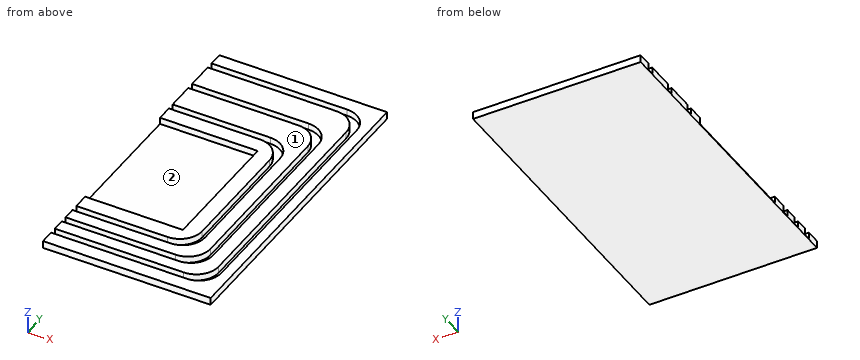
Autodesk Inventor part; units mm, degrees
ref_plane "YZ Plane" through (0, 0, 0) normal (1, 0, 0) x (0, 1, 0)
sketch "Sketch1" plane through (0, 0, 0) normal (0, 0, 1) x (1, 0, 0)
  line L0 (0, -9.3) -> (385, -9.3)
  line L1 (400, -24.3) -> (400, -185)
  line L2 (385, -200) -> (-400, -200)
  line L3 (-400, -200) -> (-400, -32.4)
  line L4 (0, -9.3) -> (0, -13.8)
  line L5 (0, -13.8) -> (380.5, -13.8)
  line L6 (395.5, -28.8) -> (395.5, -180.5)
  line L7 (380.5, -195.5) -> (-395.5, -195.5)
  line L8 (-400, -32.4) -> (372.25, -32.4)
  line L9 (387.25, -47.4) -> (387.25, -172.25)
  line L10 (372.25, -187.25) -> (-387.25, -187.25)
  line L11 (-395.5, -195.5) -> (-395.5, -36.9)
  line L12 (-395.5, -36.9) -> (367.75, -36.9)
  line L13 (382.75, -51.9) -> (382.75, -167.75)
  line L14 (367.75, -182.75) -> (-382.75, -182.75)
  line L15 (-382.75, -182.75) -> (-382.75, -60)
  line L16 (-387.25, -187.25) -> (-387.25, -55.5)
  line L17 (-387.25, -55.5) -> (359.5, -55.5)
  line L18 (374.5, -70.5) -> (374.5, -159.5)
  line L19 (-382.75, -60) -> (355, -60)
  line L20 (370, -75) -> (370, -155)
  line L21 (-561.3296, 0) -> (567.9776, 0)
  line L22 (355, -170) -> (-374.5, -170)
  line L23 (359.5, -174.5) -> (-374.5, -174.5)
  line L24 (-374.5, -174.5) -> (-374.5, -170)
  arc A0 (400, -24.3) -> (385, -9.3) centre (385, -24.3) ccw
  arc A1 (395.5, -28.8) -> (380.5, -13.8) centre (380.5, -28.8) ccw
  arc A2 (387.25, -47.4) -> (372.25, -32.4) centre (372.25, -47.4) ccw
  arc A3 (382.75, -51.9) -> (367.75, -36.9) centre (367.75, -51.9) ccw
  arc A4 (374.5, -70.5) -> (359.5, -55.5) centre (359.5, -70.5) ccw
  arc A5 (370, -75) -> (355, -60) centre (355, -75) ccw
  arc A6 (355, -170) -> (370, -155) centre (355, -155) ccw
  arc A7 (359.5, -174.5) -> (374.5, -159.5) centre (359.5, -159.5) ccw
  arc A8 (367.75, -182.75) -> (382.75, -167.75) centre (367.75, -167.75) ccw
  arc A9 (372.25, -187.25) -> (387.25, -172.25) centre (372.25, -172.25) ccw
  arc A10 (380.5, -195.5) -> (395.5, -180.5) centre (380.5, -180.5) ccw
  arc A11 (385, -200) -> (400, -185) centre (385, -185) ccw
  line L25 (406.648, 0) -> (293.548, 0)
  line L26 (293.548, 0) -> (293.548, -209.55)
  line L27 (293.548, -209.55) -> (406.648, -209.55)
  line L28 (406.648, -209.55) -> (406.648, 0)
  line L29 (293.548, -70.5) -> (359.5, -70.5)
  line L30 (359.5, -70.5) -> (359.5, -159.5)
  line L31 (359.5, -159.5) -> (293.548, -159.5)
  line L32 (293.548, -159.5) -> (293.548, -70.5)
  point P0 (0, 0)
  point P1 (400, -9.3)
  point P2 (400, -200)
  point P3 (395.5, -13.8)
  point P4 (395.5, -195.5)
  point P5 (387.25, -32.4)
  point P6 (387.25, -187.25)
  point P7 (382.75, -36.9)
  point P8 (382.75, -182.75)
  point P9 (374.5, -55.5)
  point P10 (374.5, -174.5)
  point P11 (370, -60)
  point P12 (370, -170)
  point P13 (0, 0)
  point P14 (293.548, -200)
  point P15 (293.548, 0)
  point P16 (293.548, -9.3)
  point P17 (293.548, -13.8)
  point P18 (293.548, -32.4)
  point P19 (293.548, -187.25)
  point P20 (293.548, -195.5)
  point P21 (293.548, -36.9)
  point P22 (293.548, -55.5)
  point P23 (293.548, -174.5)
  point P24 (293.548, -182.75)
  point P25 (293.548, -60)
  point P26 (293.548, -170)
  dimension "d1" = 4.5
  dimension "d2" = 4.5
  dimension "d3" = 4.5
  dimension "d4" = 9.3
  dimension "d5" = 800
  dimension "d6" = 400
  dimension "d7" = 4.5
  dimension "d8" = 4.5
  dimension "d9" = 8.25
  dimension "d10" = 4.5
  dimension "d11" = 18.6
  dimension "d12" = 4.5
  dimension "d13" = 8.25
  dimension "d14" = 4.5
  dimension "d15" = 4.5
  dimension "d16" = 4.5
  dimension "d17" = 8.25
  dimension "d19" = 18.6
  dimension "d20" = 8.25
  dimension "d82" = 200
  dimension "d88" = 4.5
  dimension "d89" = 8.25
  dimension "d90" = 8.25
  dimension "d91" = 15
  dimension "d100" = 113.1
  dimension "d101" = 209.55
extrude "Extrusion1" add sketch "Sketch1" along normal blind 4.5 contours L26 L21 L28 L27 L2 A11 L1 A0 L0 | L5 A1 L6 A10 L7 L26 L10 A9 L9 A2 L8 | L12 A3 L13 A8 L14 L26 L23 A7 L18 A4 L17 | L19 A5 L20 A6 L22 L26 L31 L30 L29
ref_plane "basePlane" through (0, 0, 0) normal (0, 0, -1) x (-1, 0, 0)
sketch "Sketch5" plane through (0, 0, 0) normal (0, 0, -1) x (-1, 0, 0)
  line L0 (-406.648, 0) -> (-293.548, 0)
  line L1 (-406.648, -209.55) -> (-406.648, 0)
  line L2 (-293.548, 0) -> (-406.648, 0)
  line L3 (-406.648, 0) -> (-406.648, -209.55)
  line L4 (-406.648, -209.55) -> (-293.548, -209.55)
  line L5 (-293.548, -209.55) -> (-293.548, 0)
  point P0 (0, 0)
extrude "Extrusion5" add sketch "Sketch5" along normal blind 0.45
equation "\"d1\" = wire_diameter"
equation "\"d2\" = wire_diameter"
equation "\"d3\" = wire_diameter"
equation "\"d4\" = 0.5 * distance_between_wires"
equation "\"d5\" = track_length"
equation "\"d7\" = wire_diameter"
equation "\"d8\" = wire_diameter"
equation "\"d9\" = distance_between_wires_edge"
equation "\"d10\" = wire_diameter"
equation "\"d11\" = distance_between_wires"
equation "\"d12\" = wire_diameter"
equation "\"d13\" = distance_between_wires_edge"
equation "\"d14\" = wire_diameter"
equation "\"d15\" = wire_diameter"
equation "\"d16\" = wire_diameter"
equation "\"d17\" = distance_between_wires_edge"
equation "\"d19\" = distance_between_wires"
equation "\"d20\" = distance_between_wires_edge"
equation "\"d82\" = 0.5 * track_width"
equation "\"d22\" = wire_diameter"
equation "\"track_length\" = 800"
equation "\"wire_diameter\" = 4.5"
equation "\"distance_between_wires\" = -1.2 * wire_diameter + 0.2 * parameter_6"
equation "\"distance_between_wires_edge\" = 8.25"
equation "\"bend_radius\" = 15"
properties part number "primary_coil_0R2"
CAD build for the part. Positions are in the model's coordinates, mm. Face numbers are marked on the shaded views. Coordinates: 2 decimals unless noted, no trailing zeros. Order: outer loops, then holes, each group sorted by start corner. A loop starts at its lowest first (then second) coordinate and runs counter-clockwise, first axis right, second up. Notation, with made-up numbers: (86, -39.5) - (130, -39.5) arc R15 ccw to (130, -10.5) - close; hole circle Ø6 at (24, -12). An arc over 180 degrees is marked (long way). Use a Markdown table: item, result. Add a question column.
(1) Saw through at C-C (z = 2.2). Count the separate pieces of the cut face and the enclosed holes in it, then the cut area to 3 significant figures.
(2) Saw through at D-D (y = -193.5). Give the cut face in (x, z), then the cut area to 3 significant figures.
(3) Flat gauge pins, fed straight in: pin 1 (10 mm diameter, centred on x = 310, y = -96, fed in from +Z); pin 2 (1.3 mm diameter, centred on x = 336, z = 3.5, fed in from +Y); pin 3 (1.3 mm diameter, centred on y = -87, z = 1.5, fed in from -X). Where does each tip first touch, or does it go through?
(4) Pull direction Y, two halves, no side cores. Call the marked faces 1 and 2: +Y half, -Y half, draft (parallel to the pull), parting line (faces both ways), or undercut.
(5) Saw through at B-B (y = -128.5). Give the cut face in (x, z), then the cut area to 3 significant figures.
(6) Drill centre lines: line 1 along X through (y, z) = (-138, 1.65); line 2 along X through (y, z) = (-54.5, 1.3); line 3 along X through (y, z) = (-176, 0.85). Where is each one in solid material? Low to high. Write a range as [from, to].
Solved:
| question | item | result |
|---|---|---|
| 1 | separate pieces | 4 |
| 1 | enclosed holes | 0 |
| 1 | area | 13,300 mm² |
| 2 | outline | (293.55, -0.45) - (406.65, -0.45) - (406.65, 4.5) - (397.36, 4.5) - (397.36, 0) - (387.98, 0) - (387.98, 4.5) - (293.55, 4.5) - close |
| 2 | area | 518 mm² |
| 3 | pin 1 | stops at z = 0 |
| 3 | pin 2 | stops at y = 0 |
| 3 | pin 3 | stops at x = 359.5 |
| 4 | face 1 | draft |
| 4 | face 2 | undercut |
| 5 | outline | (293.55, -0.45) - (406.65, -0.45) - (406.65, 4.5) - (400, 4.5) - (400, 0) - (395.5, 0) - (395.5, 4.5) - (387.25, 4.5) - (387.25, 0) - (382.75, 0) - (382.75, 4.5) - (374.5, 4.5) - (374.5, 0) - (370, 0) - (370, 4.5) - (359.5, 4.5) - (359.5, 0) - (293.55, 0) - close |
| 5 | area | 202 mm² |
| 6 | line 1 | x = [359.5, 370], [374.5, 382.75], [387.25, 395.5], [400, 406.65] |
| 6 | line 2 | x = [293.55, 382.75], [387.25, 395.5], [400, 406.65] |
| 6 | line 3 | x = [293.55, 380.28], [386.77, 395.5], [400, 406.65] |
